Here's how the part is built. I have some questions about the finished solid (model axes, mm). A direction names the side the tool comes from. Give positions to 0.01 mm unless a question says otherwise; leave off trailing zeros. Loops run counter-clockwise (first coordinate to the right, second up) from the corner with the lowest first, then second, coordinate; pieces in that order, holes last. Notation, with made-up numbers: M 88,47.25 L 115,47.25 A29 ccw 115,80.25 Z; hole C 62,-6 d11. An arc over 180 degrees is marked long. Answer as CSV lines item,"result". Start each with the question number.
Item 1: If I drill on line 1 along Z through (x, y) = (20.32, -5.5); line 2 along Z through (x, y) = (5.08, -9.5); line 3 along X through (y, z) = (-8, 3.25), over which ranges is the centre line in solid material (lowest first)? Write a range as from..to.
Item 2: For faces 4 (the cylindrical face through (6.574, -9.534, 6.915)), 5 (the flat face through (7.95, -8.53, 9.77)), 6 (the flat face through (0, -5, 10)), which set-ups out of +Z, -Z, +X, -X, +Y, -Y let a thin tool reach every point of the face, with its end or its side?
Item 3: Will these pins go through, and if not, where does the flat tip stop? P1, Ø3, axis at x = 8.5, z = 2.5, coming from the +Y side; P2, Ø1.7, axis at x = 4.5, z = 5.5, coming from the -Y side.
Item 4: I want a section at C-C on z = 12. List the corners of the cut face in (x, y) for me.
Item 5: If we mould it in two halves opening along Z, with no side actions, what happens to faces 1 (the flat face through (25.4, -5, 10)), 2 (the cylindrical face through (12.88, -1.24, 5.59)), 3 (the flat face through (13, -6, 19.812))? For each: released by +Z, released by -Z, zero draft, split by the parting line, or undercut.
Item 6: I want a section at A-A on x = 5.08. List the corners of the cut face in (y, z) for me.
Item 7: I want a section at D-D on z = 1.5. List the corners of the cut face in (x, y) for me, plus the area to 3 significant figures.
Item 8: I want a section at B-B on y = -4.75. List the corners of the cut face in (x, z) for me, plus the area to 3 significant figures.
from build123d import *

# Parameters (mm, degrees)
F0_W           = 25.4
F0_H           = 19.812
F1_DEPTH       = 10.16
F3_D           = 3.571875
F3_CBORE_D     = 5.55625
F3_CBORE_DEPTH = 1.27
F4_D           = 3.571875
F4_CBORE_D     = 5.55625
F4_CBORE_DEPTH = 1.27
F6_DEPTH       = 19.813
F8_D           = 3.048
F10_DEPTH      = 25.4


with BuildPart() as f1:
    # F0 (on Front) → F1 (new body)
    with BuildSketch(Plane.XZ):
        with Locations((12.7, 9.906)):
            Rectangle(F0_W, F0_H)
    extrude(amount=F1_DEPTH)

    # F3 (through all)
    with Locations(Plane.XZ.offset(10.16)):
        with Locations((5.08, 4.572)):
            CounterBoreHole(F3_D / 2, F3_CBORE_D / 2, F3_CBORE_DEPTH)

    # F4 (through all)
    with Locations(Plane.XZ.offset(10.16)):
        with Locations((20.32, 4.572)):
            CounterBoreHole(F4_D / 2, F4_CBORE_D / 2, F4_CBORE_DEPTH)

    # F5 (on face) → F6 (cut, through all)
    with BuildSketch(Plane(origin=(0, 0, 0), x_dir=(1, 0, 0), z_dir=(0, 0, -1))):
        Polygon((16.5071788223, 10.16), (8.89, 10.16), (6.9835894111, 6.858), (18.4135894111, 6.858), align=None)
    extrude(amount=-F6_DEPTH, mode=Mode.SUBTRACT)

    # F8 (through all)
    with Locations(Plane.XY.offset(19.812)):
        with Locations((12.6985894111, -3.8099997389)):
            Hole(F8_D / 2)

    # F9 (on face) → F10 (cut)
    with BuildSketch(Plane.YZ.offset(25.4)):
        with BuildLine():
            ThreePointArc((31.623, 4.572), (15.1765, 21.0185), (-1.27, 4.572))
            Line((-1.27, 4.572), (0, 4.572))
            Line((0, 4.572), (31.623, 4.572))
        make_face()
        with BuildLine():
            Line((0, 4.572), (-1.27, 4.572))
            ThreePointArc((-1.27, 4.572), (15.1765, -11.8745), (31.623, 4.572))
            Line((31.623, 4.572), (0, 4.572))
        make_face()
    extrude(amount=-F10_DEPTH, mode=Mode.SUBTRACT)


solid = f1.part
Result:
1,line 1,"0..2.79, 6.36..19.81"
1,line 2,"0..1.79, 7.35..19.81"
1,line 3,"0..3.88, 6.28..7.64, 17.75..19.12, 21.52..25.4"
2,face 4,"-Y"
2,face 5,"+Z, -Z"
2,face 6,"+Z, -Z, -X, +Y, -Y"
3,P1,"y = -0.88"
3,P2,"y = -8.89"
4,outline,"M 0,-10.16 L 8.89,-10.16 L 6.98,-6.86 L 18.41,-6.86 L 16.51,-10.16 L 25.4,-10.16 L 25.4,0 L 0,0 Z; hole C 12.7,-3.81 d3.05"
5,face 1,"zero draft"
5,face 2,"undercut"
5,face 3,"released by +Z"
6,outline,"M -10.16,0 L -0.62,0 A16.45 cw -1.17,2.79 L -8.89,2.79 L -8.89,1.79 L -10.16,1.79 Z; M -10.16,7.35 L -8.89,7.35 L -8.89,6.36 L -1.17,6.36 A16.45 cw 0,10.91 L 0,19.81 L -10.16,19.81 Z"
7,outline,"M 0,-10.16 L 8.89,-10.16 L 6.98,-6.86 L 18.41,-6.86 L 16.51,-10.16 L 25.4,-10.16 L 25.4,-0.98 L 0,-0.98 Z; hole C 12.7,-3.81 d3.05"
7,area,"194 mm^2"
8,outline,"M 0,0 L 11.5,0 L 11.5,19.81 L 0,19.81 Z; M 13.9,0 L 25.4,0 L 25.4,19.81 L 13.9,19.81 Z; hole C 5.08,4.57 d3.57; hole C 20.32,4.57 d3.57"
8,area,"436 mm^2"
